```python
from build123d import *

# Parameters (mm, degrees)
F0_R     = 44
F0_R_2   = 1.65
F1_DEPTH = 3


with BuildPart() as f1:
    # F0 (on Top) → F1 (new body)
    with BuildSketch(Plane.XY):
        Circle(F0_R)
        with Locations((0, -39.064214)):
            Circle(F0_R_2, mode=Mode.SUBTRACT)
        with Locations((-33.830601, 19.532107)):
            Circle(F0_R_2, mode=Mode.SUBTRACT)
        with BuildLine():
            Line((5.1, 34.800884), (5.1, 25))
            Line((5.1, 25), (10, 25))
            ThreePointArc((10, 25), (20.606602, 20.606602), (25, 10))
            Line((25, 10), (25, -10))
            ThreePointArc((25, -10), (20.606602, -20.606602), (10, -25))
            Line((10, -25), (-10, -25))
            ThreePointArc((-10, -25), (-20.606602, -20.606602), (-25, -10))
            Line((-25, -10), (-25, 10))
            ThreePointArc((-25, 10), (-20.606602, 20.606602), (-10, 25))
            Line((-10, 25), (-5.1, 25))
            Line((-5.1, 25), (-5.1, 34.800884))
            Line((-5.1, 34.800884), (5.1, 34.800884))
        make_face(mode=Mode.SUBTRACT)
        with Locations((33.830601, 19.532107)):
            Circle(F0_R_2, mode=Mode.SUBTRACT)
    extrude(amount=F1_DEPTH)


solid = f1.part
```
Geometry check sheet. Reference: the model listing, model coordinates, mm. A direction names the side the tool comes from. Give positions to 0.01 mm unless a question says otherwise; leave off trailing zeros. Loops run counter-clockwise (first coordinate to the right, second up) from the corner with the lowest first, then second, coordinate; pieces in that order, holes last. Notation, with made-up numbers: M 35.25,53 L 62.25,53 A13 cw 62.25,57 Z; hole C -20.5,54.25 d2. An arc over 180 degrees is marked long. Write item = value, one per line.
(1) Sectioned sample at A-A, the plane x = 0. Record the cut outline in (y, z).
Answer below:
outline = M -44,0 L -40.71,0 L -40.71,3 L -44,3 Z; M -37.41,0 L -25,0 L -25,3 L -37.41,3 Z; M 34.8,0 L 44,0 L 44,3 L 34.8,3 Z
(2) Sectioned sample at C-C, the plane x = -15.5. Record the cut outline in (y, z).
Answer below:
outline = M -41.18,0 L -23.96,0 L -23.96,3 L -41.18,3 Z; M 23.96,0 L 41.18,0 L 41.18,3 L 23.96,3 Z
(3) Sectioned sample at B-B, the plane y = 0. Record the cut outline in (x, z), plus the area to 3 significant figures.
Answer below:
outline = M -44,0 L -25,0 L -25,3 L -44,3 Z; M 25,0 L 44,0 L 44,3 L 25,3 Z
area = 114 mm2
(4) Gauge pin test, flat ends, axial feed: pin 1 Ø0.9 at (y, z) = (30.5, 2) entering from -X; pin 2 Ø1.5 at (x, y) = (12.5, -23) entering from +Z; pin 3 Ø0.9 at (y, z) = (2, 2) entering from -X; pin 4 Ø0.9 at (x, z) = (-7, 2) entering from -Y. Record the tip position at first contact, or that the pin passes through.
Answer below:
pin_1 = -32.14
pin_2 = through
pin_3 = -43.97
pin_4 = -43.51
(5) Material ranges on line 1 (Y direction, x = 0, z = 0.7); line 2 (X direction, y = -1, z = 1.6); line 3 (X direction, y = -6.5, z = 1.6), recorded low to high. Write a range as [from, to].
Answer below:
line_1 = [-44, -40.71], [-37.41, -25], [34.8, 44]
line_2 = [-43.99, -25], [25, 43.99]
line_3 = [-43.52, -25], [25, 43.52]
(6) Sectioned sample at D-D, the plane z = 1.2. Record the cut outline in (x, y), plus the area to 3 significant figures.
Answer below:
outline = C 0,0 d88; hole C -33.83,19.53 d3.3; hole M -25,-10 A15 ccw -10,-25 L 10,-25 A15 ccw 25,-10 L 25,10 A15 ccw 10,25 L 5.1,25 L 5.1,34.8 L -5.1,34.8 L -5.1,25 L -10,25 A15 ccw -25,10 Z; hole C 0,-39.06 d3.3; hole C 33.83,19.53 d3.3
area = 3,650 mm2
(7) Release check for a two-part mould opening along X. For faces 3 (the face through (20.72, -20.49, 1.48)), 4 (the face through (-9.538, -42.954, 1.479)), 5 (the face through (29, 1, 0)) record: released by +X, released by -X, zero draft, split by the parting line, or undercut.
Answer below:
face_3 = undercut
face_4 = split by the parting line
face_5 = zero draft
(8) Tool access check on faces 1 (the face through (29, 1, 3)), 2 (the face through (-20.49, -20.72, 1.48)). Record the directions out of +Z, -Z, +X, -X, +Y, -Y that give a thin tool (end or side, any length) a straight path to the whole face; none if there is none.
Answer below:
face_1 = +Z, +X, -X, +Y, -Y
face_2 = +Z, -Z
